Work out the finished part from the listing and answer in its coordinate system (mm). A direction names the side the tool comes from. Give positions to 0.01 mm unless a question says otherwise; leave off trailing zeros. Loops run counter-clockwise (first coordinate to the right, second up) from the corner with the lowest first, then second, coordinate; pieces in that order, holes last. Notation, with made-up numbers: M -6.5,-39 L 2.5,-39 A24 ccw 2.5,-23 Z; hole C 46.25,77 d2. An arc over 180 degrees is marked long. Use a Markdown table: item, result.
```python
from build123d import *

# Parameters (mm, degrees)
SALIENTE_EXTRUIR1_DEPTH   = 8
CROQUIS1_W                = 2.4
CROQUIS1_H                = 7.15885354
SALIENTE_EXTRUIR1_2_DEPTH = 8
CROQUIS2_W                = 5.5
CROQUIS2_H                = 7.15885354
SALIENTE_EXTRUIR2_DEPTH   = 1.5
CROQUIS3_W                = 5.5
CROQUIS3_H                = 2.15885354
CORTAR_EXTRUIR1_DEPTH     = 10.5


with BuildPart() as part:
    # Croquis1 → Saliente-Extruir1 (new body)
    with BuildSketch(Plane.XY):
        Polygon((0, 7.15885354), (0, 6.4), (0.6, 6.3), (0.6, 5.1), (0, 5), (0, 4.279426768), (0.6, 4.179426768), (0.6, 2.979426768), (0, 2.879426768), (0, 2.158853536), (0.6, 2.058853536), (0.6, 0.858853536), (0, 0.758853536), (0, 0), (2.4, 0), (2.4, 7.15885354), align=None)
    extrude(amount=SALIENTE_EXTRUIR1_DEPTH)



with BuildPart() as body_2:
    # Croquis1 → Saliente-Extruir1 2 (new body)
    with BuildSketch(Plane.XY):
        with Locations((-1.9, 3.57942677)):
            Rectangle(CROQUIS1_W, CROQUIS1_H)
    extrude(amount=SALIENTE_EXTRUIR1_2_DEPTH)


with BuildPart() as part_1:
    add(part.part)

    add(body_2.part)  # Saliente-Extruir2 merges body 2
    # Croquis2 → Saliente-Extruir2 (add)
    with BuildSketch(Plane(origin=(0, 0, 0), x_dir=(-1, 0, 0), z_dir=(0, 0, -1))):
        with Locations((0.35, 3.57942677)):
            Rectangle(CROQUIS2_W, CROQUIS2_H)
    extrude(amount=SALIENTE_EXTRUIR2_DEPTH)

    # Croquis3 → Cortar-Extruir1 (cut, through all)
    with BuildSketch(Plane.XY.offset(8)):
        with Locations((-0.35, 6.07942677)):
            Rectangle(CROQUIS3_W, CROQUIS3_H)
    extrude(amount=-CORTAR_EXTRUIR1_DEPTH, mode=Mode.SUBTRACT)


solid = part_1.part
```
(1) A cutting plane is placed at B-B (y = 0.6). Write down the section's boundary in (x, z), and give its area (4 significant figures).
Entries:
| item | result |
|---|---|
| outline | M -3.1,-1.5 L 2.4,-1.5 L 2.4,8 L 0,8 L 0,0 L -0.7,0 L -0.7,8 L -3.1,8 Z |
| area | 46.65 mm² |
(2) Which of the six approach directions +Z, -Z, +X, -X, +Y, -Y give full straight-line access (tool end or side, diameter ignored) to faces 4 (the flat face through (0.6, 1.5, 3.9)), 5 (the flat face through (0, 3, -1.5)), 6 (the flat face through (-0.7, 2, 4))?
Entries:
| item | result |
|---|---|
| face 4 | +Z |
| face 5 | -Z, +X, -X, +Y, -Y |
| face 6 | +Z, +Y, -Y |
(3) Consider probe 1 along X at (y, z) = (1.25, 2.5); probe 2 along X at (y, z) = (4.75, 4); probe 3 along Z at (x, y) = (0.25, 1.85). Determine where each line is inside the solid, lowest interval first. Write a range as [from, to].
Entries:
| item | result |
|---|---|
| probe 1 | x = [-3.1, -0.7], [0.6, 2.4] |
| probe 2 | x = [-3.1, -0.7], [0, 2.4] |
| probe 3 | z = [-1.5, 0] |
(4) A cutting plane is placed at C-C (y = 1.35). Write down the section's boundary in (x, z), and give its area (4 significant figures).
Entries:
| item | result |
|---|---|
| outline | M -3.1,-1.5 L 2.4,-1.5 L 2.4,8 L 0.6,8 L 0.6,0 L -0.7,0 L -0.7,8 L -3.1,8 Z |
| area | 41.85 mm² |
(5) A cutting plane is placed at A-A (z = 0.5). Write down the section's boundary in (x, y), and give its area (3 significant figures).
Entries:
| item | result |
|---|---|
| outline | M -3.1,0 L -0.7,0 L -0.7,5 L -3.1,5 Z; M 0,0 L 2.4,0 L 2.4,5 L 0,5 L 0,4.28 L 0.6,4.18 L 0.6,2.98 L 0,2.88 L 0,2.16 L 0.6,2.06 L 0.6,0.86 L 0,0.76 Z |
| area | 22.4 mm² |
(6) The mould has two halves that part along X. Classify faces 1 (the flat face through (-0.2, 2.5, 0)), 2 (the flat face through (2.4, 2, 3)), 3 (the flat face through (-1, 5, 3)): released by +X, released by -X, zero draft, split by the parting line, or undercut.
Entries:
| item | result |
|---|---|
| face 1 | undercut |
| face 2 | released by +X |
| face 3 | zero draft |
